```python
from build123d import *

# Parameters (mm, degrees)
SKETCH1_R      = 1.4
EXTRUDE1_DEPTH = 5.5


# Read off the part's stored shape, not the designer's step: Cut-Extrude1
with BuildPart() as part:
    # Sketch1 → Extrude1 (new, symmetric)
    with BuildSketch(Plane(origin=(0, 0, 0), x_dir=(0, 0, -1), z_dir=(1, 0, 0))):
        Polygon((2.696225757, 0), (1.348112879, 2.335), (-1.348112879, 2.335), (-2.696225757, 0), (-1.348112879, -2.335), (1.348112879, -2.335), align=None)
        Circle(SKETCH1_R, mode=Mode.SUBTRACT)
    extrude(amount=EXTRUDE1_DEPTH, both=True)

    # Cut-Extrude1 outline → Cut-Extrude1 (revolve, cut)
    with BuildSketch(Plane.YX):
        Polygon((2.696225758, 5.5), (2.335, 5.5), (2.696225751, 5.291446215), align=None)
    cut_extrude1 = revolve(axis=Axis((0, 0, 0), (1, 0, 0)), mode=Mode.SUBTRACT)

    # Mirror1: Cut-Extrude1 across plane
    add(cut_extrude1.mirror(Plane(origin=(0, 0, 0), x_dir=(0, 0, 1), z_dir=(1, 0, 0))), mode=Mode.SUBTRACT)


solid = part.part
```
The model under review builds one solid part; all positions refer to its coordinate system, in mm. Round coordinates to 2 decimals unless told otherwise and drop trailing zeros. Order: outer loops, then holes, each group sorted by start corner. A loop starts at its lowest first (then second) coordinate and runs counter-clockwise, first axis right, second up. Notation, with made-up numbers: (-25, 72.25) -> (-15, 72.25) arc R14 ccw to (-15, 88.25) -> close; hole circle Ø4 at (89.25, 67.25). An arc over 180 degrees is marked (long way). One line per item, written item: value. Start each with the question number.
Q1. Take a section at A-A (x = 1.5). Write out the cut boundary in (y, z) (3 decimals), and give its area (3 significant figures).
Q2. Clearance check with flat-ended pins moving along their axes: pin 1 Ø1 at (x, z) = (-2.5, -2) entering from -Y; pin 2 Ø2 at (x, y) = (2, 2) entering from +Z. State where each tip first meets the part, or that it passes through.
Q3. Wall thickness on line 1 (Y direction, x = 0.25, z = 0) (3 decimals); line 2 (Y direction, x = -3.5, z = 0.9) (3 decimals); line 3 (Z direction, x = 1.5, y = -0.7): over which ranges is each line inside the solid? List them lowest first.
Q4. Mouldability with a two-part tool opening along Y and no side actions: class faces 1 (the face through (0, -2.335, 0)), 2 (the face through (5.4, 2.2, 1.2)), 3 (the face through (-0.08, 0.06, 1.4)) as released by +Y, released by -Y, zero draft, split by the parting line, or undercut.
Reported:
1. outline: (-2.335, -1.348) -> (0, -2.696) -> (2.335, -1.348) -> (2.335, 1.348) -> (0, 2.696) -> (-2.335, 1.348) -> close; hole circle Ø2.8 at (0, 0)
1. area: 12.7 mm2
2. pin 1: stops at y = -2.07
2. pin 2: stops at z = 2.12
3. line 1: y = -2.335 to -1.4, 1.4 to 2.335
3. line 2: y = -2.335 to -1.072, 1.072 to 2.335
3. line 3: z = -2.29 to -1.21, 1.21 to 2.29
4. face 1: released by -Y
4. face 2: released by +Y
4. face 3: undercut
